Geometry: final body of the model. Coordinates: model frame, mm. A direction names the side the tool comes from. Give positions to 0.01 mm unless a question says otherwise; leave off trailing zeros. Loops run counter-clockwise (first coordinate to the right, second up) from the corner with the lowest first, then second, coordinate; pieces in that order, holes last. Notation, with made-up numbers: (-3.5, -20) -> (26.5, -20) arc R19 ccw to (26.5, 6) -> close; hole circle Ø4 at (89.25, -12). An arc over 180 degrees is marked (long way). Answer in a Markdown table with one row per item. Add a question column.
1) First-contact query: P1, Ø1.5, axis at x = 20, z = 29, coming from the +Y side; P2, Ø12, axis at y = 1.5, z = -17, coming from the -X side; P3, Ø4, axis at x = 28.5, y = 8, coming from the +Z side; P4, Ø7, axis at x = -46.72, z = -46.72, coming from the -Y side. Flat tips, straight axial feed; report the tip coordinate or a pass-through.
2) Section query A-A (y = -13.5). Return the cut outline in (x, z), plus the area to 3 significant figures.
3) Access query for faces 5 (the flat face through (-20, 12.62, -28)), 6 (the flat face through (-36.32, -13.8, -36.57)), 7 (the flat face through (-31, 15, 25)), 8 (the flat face through (29, 21, 23.46)). Directions: +Z, -Z, +X, -X, +Y, -Y. A direction counts if a zero-diameter tool reaches every point of the face in a straight line with its end or side. Return the directions, or none.
4) Section query B-B (z = -54). Return the cut outline in (x, y), plus the area to 3 significant figures.
5) Line query: line 1 (X direction, y = 15, z = 24); line 2 (X direction, y = 16, z = -29.5); line 3 (Y direction, x = -26, z = 7). Output: solid intervals per line, ascending. Write a range as from..to.
6) Section query C-C (y = 1.5). Return the cut outline in (x, z).
7) Draft query along Z for faces 1 (the flat face through (-25, 15, 31)), 2 (the flat face through (-45.72, -11.58, 27.76)), 3 (the flat face through (-43, -28, -43)), 4 (the flat face through (29, 9, 16)). Return one class per face: +Z half, -Z half, draft (parallel to the pull), parting line (faces both ways), or undercut.
8) Section query D-D (x = 29). Return the cut outline in (y, z), plus the area to 3 significant figures.
```python
from build123d import *

# Parameters (mm, degrees)
BOSS_EXTRUDE1_DEPTH = 5
BOSS_EXTRUDE2_DEPTH = 7.62
BOSS_EXTRUDE3_DEPTH = 28
SKETCH5_W           = 25.4
SKETCH5_H           = 5
BOSS_EXTRUDE4_DEPTH = 19.05
SKETCH6_W           = 25.4
SKETCH6_H           = 5
BOSS_EXTRUDE5_DEPTH = 19.05
SKETCH7_W           = 25.4
SKETCH7_H           = 5
BOSS_EXTRUDE6_DEPTH = 19.05
SKETCH8_W           = 25.4
SKETCH8_H           = 5
BOSS_EXTRUDE7_DEPTH = 19.05
SKETCH9_R           = 4.5
CUT_EXTRUDE1_DEPTH  = 12.7
BOSS_EXTRUDE8_DEPTH = 25.4


with BuildPart() as part:
    # Sketch2 → Boss-Extrude1 (new body)
    with BuildSketch(Plane(origin=(0, 0, 0), x_dir=(1, 0, 0), z_dir=(0, 1, 0))):
        Polygon((-48.960512242, 31), (-26.509871939, 8.549359697), (-26.509871939, -8.549359697), (-48.960512242, -31), (-31, -48.960512242), (-8.549359697, -26.509871939), (8.549359697, -26.509871939), (31, -48.960512242), (48.960512242, -31), (26.509871939, -8.549359697), (26.509871939, 8.549359697), (48.960512242, 31), (31, 48.960512242), (8.549359697, 26.509871939), (-8.549359697, 26.509871939), (-31, 48.960512242), align=None)
    extrude(amount=BOSS_EXTRUDE1_DEPTH)

    # Sketch3 → Boss-Extrude2 (add)
    with BuildSketch(Plane(origin=(0, 5, 0), x_dir=(-1, 0, 0), z_dir=(0, 1, 0))):
        Polygon((31, 31), (16, 31), (16, 26), (26, 26), (26, 16), (31, 16), align=None)
        Polygon((31, -31), (31, -16), (26, -16), (26, -26), (16, -26), (16, -31), align=None)
        Polygon((-31, 31), (-31, 16), (-26, 16), (-26, 26), (-16, 26), (-16, 31), align=None)
        Polygon((-31, -31), (-16, -31), (-16, -26), (-26, -26), (-26, -16), (-31, -16), align=None)
    extrude(amount=BOSS_EXTRUDE2_DEPTH)

    # Sketch4 → Boss-Extrude3 (add)
    with BuildSketch(Plane(origin=(0, 0, 0), x_dir=(-1, 0, 0), z_dir=(0, -1, 0))):
        Polygon((31, -48.960512242), (48.960512242, -31), (45.424978336, -27.464466094), (27.464466094, -45.424978336), align=None)
        Polygon((48.960512242, 31), (31, 48.960512242), (27.464466094, 45.424978336), (45.424978336, 27.464466094), align=None)
        Polygon((-31, 48.960512242), (-48.960512242, 31), (-45.424978336, 27.464466094), (-27.464466094, 45.424978336), align=None)
        Polygon((-48.960512242, -31), (-31, -48.960512242), (-27.464466094, -45.424978336), (-45.424978336, -27.464466094), align=None)
    extrude(amount=BOSS_EXTRUDE3_DEPTH)

    # Sketch5 → Boss-Extrude4 (add)
    with BuildSketch(Plane(origin=(104.086919113, 0, 24.126406871), x_dir=(0.7071067811865459, 0, 0.7071067811865492), z_dir=(-0.7071067811865492, 0, 0.7071067811865459))):
        with Locations((-90.660512242, -25.5)):
            Rectangle(SKETCH5_W, SKETCH5_H)
    extrude(amount=-BOSS_EXTRUDE4_DEPTH)

    # Sketch6 → Boss-Extrude5 (add)
    with BuildSketch(Plane(origin=(32.44615075, 0, -112.406662992), x_dir=(0.7071067811865465, 0, -0.7071067811865487), z_dir=(0.7071067811865487, 0, 0.7071067811865465))):
        with Locations((-102.426406871, -25.5)):
            Rectangle(SKETCH6_W, SKETCH6_H)
    extrude(amount=-BOSS_EXTRUDE5_DEPTH)

    # Sketch7 → Boss-Extrude6 (add)
    with BuildSketch(Plane(origin=(-39.980256121, 0, 39.980256121), x_dir=(-0.7071067811865459, 0, -0.7071067811865492), z_dir=(0.7071067811865492, 0, -0.7071067811865459))):
        with Locations((0, -25.5)):
            Rectangle(SKETCH7_W, SKETCH7_H)
    extrude(amount=-BOSS_EXTRUDE6_DEPTH)

    # Sketch8 → Boss-Extrude7 (add)
    with BuildSketch(Plane(origin=(39.980256121, 0, 39.980256121), x_dir=(0.7071067811865459, 0, -0.7071067811865492), z_dir=(0.7071067811865492, 0, 0.7071067811865459))):
        with Locations((0, -25.5)):
            Rectangle(SKETCH8_W, SKETCH8_H)
    extrude(amount=BOSS_EXTRUDE7_DEPTH)

    # Sketch9 → Cut-Extrude1 (cut)
    with BuildSketch(Plane(origin=(0, -23, 0), x_dir=(1, 0, 0), z_dir=(0, 1, 0))):
        with Locations(Location((46.715448212, -46.715448212, 0), (0, 0, 270))):
            Circle(SKETCH9_R)
        with Locations(Location((46.715448212, 46.715448212, 0), (0, 0, 270))):
            Circle(SKETCH9_R)
        with Locations(Location((-46.715448212, 46.715448212, 0), (0, 0, 270))):
            Circle(SKETCH9_R)
        with Locations(Location((-46.715448212, -46.715448212, 0), (0, 0, 270))):
            Circle(SKETCH9_R)
    extrude(amount=-CUT_EXTRUDE1_DEPTH, mode=Mode.SUBTRACT)

    # Sketch10 → Boss-Extrude8 (add)
    with BuildSketch(Plane(origin=(0, 5, 0), x_dir=(1, 0, 0), z_dir=(0, 1, 0))):
        Polygon((31, -31), (31, -23.46), (26, -23.46), (26, -26), (23.46, -26), (23.46, -31), align=None)
        Polygon((23.46, 31), (23.46, 26), (26, 26), (26, 23.46), (31, 23.46), (31, 31), align=None)
        Polygon((-31, 31), (-31, 23.46), (-26, 23.46), (-26, 26), (-23.46, 26), (-23.46, 31), align=None)
        Polygon((-23.46, -31), (-23.46, -26), (-26, -26), (-26, -23.46), (-31, -23.46), (-31, -31), align=None)
    extrude(amount=BOSS_EXTRUDE8_DEPTH)


solid = part.part
```
Evaluation:
| question | item | result |
|---|---|---|
| 1 | P1 | y = 12.62 |
| 1 | P2 | x = -40.96 |
| 1 | P3 | z = 31 |
| 1 | P4 | through |
| 2 | outline | (-48.96, -31) -> (-31, -48.96) -> (-27.46, -45.42) -> (-45.42, -27.46) -> close; (-48.96, 31) -> (-45.42, 27.46) -> (-27.46, 45.42) -> (-31, 48.96) -> close; (27.46, -45.42) -> (31, -48.96) -> (48.96, -31) -> (45.42, -27.46) -> close; (27.46, 45.42) -> (45.42, 27.46) -> (48.96, 31) -> (31, 48.96) -> close |
| 2 | area | 508 mm² |
| 3 | face 5 | +Z, -Z, +Y |
| 3 | face 6 | -Y |
| 3 | face 7 | +Z, -Z, -X, +Y |
| 3 | face 8 | +X, -X, +Y |
| 4 | outline | (-52.9, -28) -> (-36.04, -28) -> (-36.04, -23) -> (-52.9, -23) -> close; (36.04, -28) -> (52.9, -28) -> (52.9, -23) -> (36.04, -23) -> close |
| 4 | area | 169 mm² |
| 5 | line 1 | -31..-26, 26..31 |
| 5 | line 2 | -31..-23.46, 23.46..31 |
| 5 | line 3 | 0..5 |
| 6 | outline | (-48.96, -31) -> (-31, -48.96) -> (-8.55, -26.51) -> (8.55, -26.51) -> (31, -48.96) -> (48.96, -31) -> (26.51, -8.55) -> (26.51, 8.55) -> (48.96, 31) -> (31, 48.96) -> (8.55, 26.51) -> (-8.55, 26.51) -> (-31, 48.96) -> (-48.96, 31) -> (-26.51, 8.55) -> (-26.51, -8.55) -> close |
| 7 | face 1 | +Z half |
| 7 | face 2 | undercut |
| 7 | face 3 | draft |
| 7 | face 4 | undercut |
| 8 | outline | (-28, -46.96) -> (5, -46.96) -> (5, -31) -> (30.4, -31) -> (30.4, -23.46) -> (12.62, -23.46) -> (12.62, -16) -> (5, -16) -> (5, -11.04) -> (0, -11.04) -> (0, -43.89) -> (-28, -43.89) -> close; (-28, 43.89) -> (0, 43.89) -> (0, 11.04) -> (5, 11.04) -> (5, 16) -> (12.62, 16) -> (12.62, 23.46) -> (30.4, 23.46) -> (30.4, 31) -> (5, 31) -> (5, 46.96) -> (-28, 46.96) -> close |
| 8 | area | 1,030 mm² |
